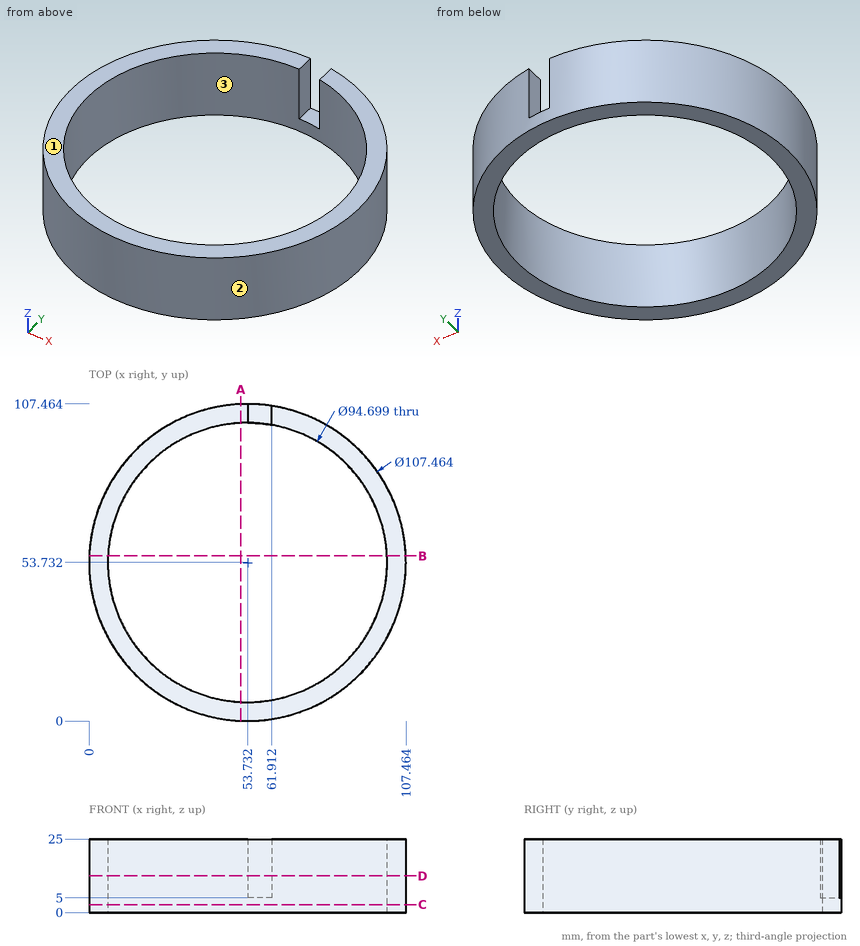
Can you work these out from the drawing? Everything is in mm from the part's minimum corner. Coordinates: 2 decimals unless noted, no trailing zeros. Write each loop counter-clockwise with the first axis right and the second up, starting at its lowest first coordinate (ties: lowest second). Pieces come first, ordered by that corner, then holes. Notation, with made-up numbers: (77.5, 52.25) -> (100.5, 52.25) arc R15 cw to (100.5, 79.25) -> close; hole circle Ø2 at (35, 84). An arc over 180 degrees is marked (long way). Write each question's results on one line, items separated by ' | '. Start each with the question number.
Q1. If I drill on probe 1 along Y at (x, z) = (23, 5.5) (1 decimal); probe 2 along Y at (x, z) = (85, 1.75) (1 decimal); probe 3 along X at (y, z) = (15, 10.75) (1 decimal), over which ranges is the centre line in solid material (lowest first)?
Q2. I'm going to push flat-ended pins straight in: pin 1 (6 mm diameter, centred on x = 16.5, z = 21.5, fed in from +Y); pin 2 (5 mm diameter, centred on x = 60.5, z = 17, fed in from +Y); pin 3 (6 mm diameter, centred on x = 73.5, z = 4.5, fed in from -Y). Where does each tip first touch, or does it pass through?
Q3. Imagine slicing it at A-A (x = 51.5). Write out the boundary of the cut face in (y, z) (1 decimal).
Q4. Imagine slicing it at C-C (z = 2.75). Write out the boundary of the cut face in (x, y).
Q5. We'd pull the mould along Y, two halves only. Please class the marked faces 1, 2 and 3: +Y half, -Y half, draft (parallel to the pull), parting line (faces both ways), or undercut.
Q6. Imagine slicing it at D-D (z = 12.5). Write out the boundary of the cut face in (x, y), then the cut area to 3 significant figures.
Taken from the geometry:
1) probe 1: y = 9.7 to 17.7, 89.8 to 97.8 | probe 2: y = 10 to 18.2, 89.3 to 97.4 | probe 3: x = 16.5 to 26.5, 81 to 91
2) pin 1: stops at y = 95.15 | pin 2: stops at y = 106.84 | pin 3: stops at y = 2.68
3) outline: (0, 0) -> (6.4, 0) -> (6.4, 25) -> (0, 25) -> close; (101, 0) -> (107.4, 0) -> (107.4, 25) -> (101, 25) -> close
4) outline: circle Ø107.46 at (53.73, 53.73); hole circle Ø94.7 at (53.73, 53.73)
5) face 1: draft | face 2: parting line | face 3: undercut
6) outline: (53.73, 101.08) -> (53.73, 107.46) arc R53.73 ccw (long way) to (61.91, 106.84) -> (61.91, 100.37) arc R47.35 cw (long way) to start | area: 1,970 mm^2
